Here's how the part is built. I have some questions about the finished solid (model axes, mm). Face numbers are marked on the shaded views. A direction names the side the tool comes from. Give positions to 0.01 mm unless a question says otherwise; leave off trailing zeros. Write each loop counter-clockwise with the first axis right and the second up, starting at its lowest first coordinate (ties: lowest second). Pieces come first, ordered by that corner, then holes. Notation, with made-up numbers: M 88,-16.5 L 111,-16.5 A18 ccw 111,15.5 Z; hole C -27,53.25 d7. An arc over 180 degrees is marked long. Use one line per item in the form item = value. Start each with the question number.
Autodesk Inventor part; units mm, degrees
ref_plane "YZ Plane" through (0, 0, 0) normal (1, 0, 0) x (0, 1, 0)
ref_plane "XZ Plane" through (0, 0, 0) normal (0, 1, 0) x (-1, 0, 0)
ref_plane "XY Plane" through (0, 0, 0) normal (0, 0, 1) x (1, 0, 0)
sketch "Sketch1" plane through (0, 0, 0) normal (0, 0, 1) x (1, 0, 0)
  circle A0 centre (0, 0) radius 2.5
  circle A1 centre (0, 0) radius 5.5
  circle A2 centre (0, 0) radius 4.75
  circle A3 centre (0, 0) radius 3.25
  dimension "d0" = 5
  dimension "d1" = 11
  dimension "d2" = 0.75
  dimension "d3" = 0.75
extrude "Extrusion1" add sketch "Sketch1" along normal mid plane 3
extrude "Extrusion2" add sketch "Sketch1" along normal mid plane 2.75 contours A2
sketch "Sketch2" plane through (0, 0, 1.5) normal (0, 0, 1) x (1, 0, 0)
  circle A0 centre (0, 0) radius 5.5
  circle A1 centre (0, 0) radius 6.25
  dimension "d8" = 12.5
extrude "Extrusion3" add sketch "Sketch2" against normal blind 0.8
properties part number "F685ZZ" material "Steel, Carbon"
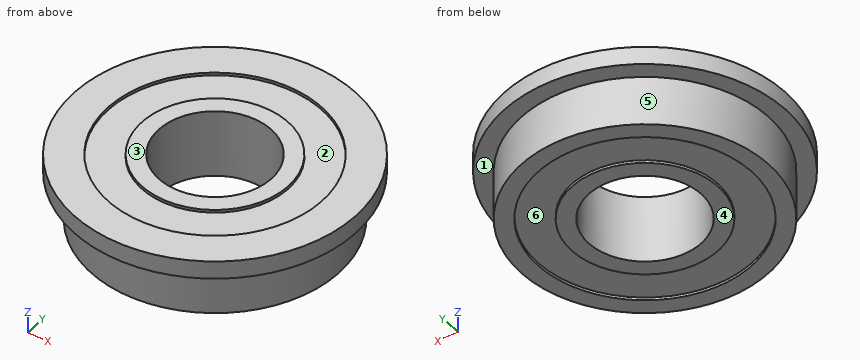
1) Suppose I cut it at A-A, the plane x = 0. List the corners of the cut face in (y, z) for me (3 decimals).
2) Suppose I cut it at C-C, the plane y = -4.5. List the corners of the cut face in (x, z) for me (3 decimals).
3) Suppose I cut it at D-D, the plane z = -0.5. List the corners of the cut face in (x, y) for me, and give its area (3 significant figures).
4) On a 3-axis mill with a long thin cutter (end or side, diameter ignored), from which of +Z, -Z, +X, -X, +Y, -Y can I reach the whole of each face in a straight line? I mean the marked faces 1, 2 and 3. Say none if no direction works.
5) Thinking about a two-plate mould opening in Y: for the marked faces 4, 5 and 6, which applies, released by +Y, released by -Y, zero draft, split by the parting line, or undercut?
6) Will these pins go through, and if not, where does the flat tip stop? P1, Ø1.5, axis at y = -3.5, z = 1, coming from the -X side; P2, Ø1, axis at y = -0.5, z = -1, coming from the +X side; P3, Ø4, axis at x = 0, y = 0, coming from the -Z side.
7) Please list where these lines run through material, in increasing order: line 1 (Y direction, x = 0, z = -0.4); line 2 (Y direction, x = 0, z = 1.45); line 3 (Z direction, x = -2.75, y = -3.5) (3 decimals).
Checks:
q1.outline = M -6.25,0.7 L -5.5,0.7 L -5.5,-1.5 L -4.75,-1.5 L -4.75,-1.375 L -3.25,-1.375 L -3.25,-1.5 L -2.5,-1.5 L -2.5,1.5 L -3.25,1.5 L -3.25,1.375 L -4.75,1.375 L -4.75,1.5 L -6.25,1.5 Z; M 2.5,-1.5 L 3.25,-1.5 L 3.25,-1.375 L 4.75,-1.375 L 4.75,-1.5 L 5.5,-1.5 L 5.5,0.7 L 6.25,0.7 L 6.25,1.5 L 4.75,1.5 L 4.75,1.375 L 3.25,1.375 L 3.25,1.5 L 2.5,1.5 Z
q2.outline = M -4.337,0.7 L -3.162,0.7 L -3.162,-1.5 L -1.521,-1.5 L -1.521,-1.375 L 1.521,-1.375 L 1.521,-1.5 L 3.162,-1.5 L 3.162,0.7 L 4.337,0.7 L 4.337,1.5 L 1.521,1.5 L 1.521,1.375 L -1.521,1.375 L -1.521,1.5 L -4.337,1.5 Z
q3.outline = C 0,0 d11; hole C 0,0 d5
q3.area = 75.4 mm^2
q4.face_1 = -Z
q4.face_2 = +Z
q4.face_3 = +Z, +X, -X, +Y, -Y
q5.face_4 = zero draft
q5.face_5 = split by the parting line
q5.face_6 = undercut
q6.P1 = -5.61
q6.P2 = 5.5
q6.P3 = through
q7.line_1 = -5.5 to -2.5, 2.5 to 5.5
q7.line_2 = -6.25 to -4.75, -3.25 to -2.5, 2.5 to 3.25, 4.75 to 6.25
q7.line_3 = -1.375 to 1.375
